Autodesk Inventor part; units mm, degrees
ref_plane "Work Plane1" through (1.525, 0, 0) normal (0, 0, 1) x (1, 0, 0)
ref_plane "YZ Plane" through (0, 0, 0) normal (1, 0, 0) x (0, 1, 0)
ref_plane "XZ Plane" through (0, 0, 0) normal (0, 1, 0) x (-1, 0, 0)
sketch "草图1" plane through (0, 0, 0) normal (0, 0, 1) x (1, 0, 0)
  line L0 (0, 7.25) -> (0, 5)
  line L1 (9, 5) -> (35, 5)
  line L2 (35, 5) -> (35, 0)
  line L3 (35, 0) -> (-0.4001, 0)
  line L4 (-7.4801, 0) -> (42.08, 0)
  line L5 (-0.4001, 0) -> (-0.4001, 7.25)
  line L6 (-0.4001, 7.25) -> (0, 7.25)
  line L7 (9, 5) -> (8.0797, 5)
  line L8 (8.0797, 5) -> (0, 5)
  line L9 (0, -1.45) -> (0, 8.7)
  dimension "d0" = 35
  dimension "d1" = 26
  dimension "d2" = 10
  dimension "d9" = 0.4001
  dimension "d10" = 14.5
  dimension "d13" = 0.9203
  dimension "d14" = 10
revolve "轴承体" add sketch "草图1" angle 360 about axis through (35, 0, 0) along (-1, 0, 0)
sketch "草图2" plane through (-0.4001, 0, 0) normal (-1, 0, 0) x (0, 0, 1)
  line L0 (0, 9.2376) -> (8, 4.6188)
  line L1 (8, 4.6188) -> (8, -4.6188)
  line L2 (8, -4.6188) -> (0, -9.2376)
  line L3 (0, -9.2376) -> (-8, -4.6188)
  line L4 (-8, -4.6188) -> (-8, 4.6188)
  line L5 (-8, 4.6188) -> (0, 9.2376)
  point P0 (0, 0)
  point P1 (0, 0)
  dimension "d11" = 16
extrude "头" add sketch "草图2" along normal blind 6
sketch "草图4" plane through (0, 0, 0) normal (0, 0, 1) x (1, 0, 0)
  line L0 (-6.4001, 8) -> (-6.4001, 9.2376)
  line L1 (-6.4001, 9.2376) -> (-5.6856, 9.2376)
  line L2 (-5.6856, 9.2376) -> (-6.4001, 8)
  line L3 (-7.6001, 0) -> (0.7999, 0)
  line L4 (-0.4001, 9.2376) -> (-6.4001, 9.2376)
  line L5 (-6.4001, 4.6188) -> (-6.4001, 9.2376)
  dimension "d5" = 30
  dimension "d19" = 16
revolve "倒角1" cut sketch "草图4" angle 360 about axis through (-10, 0, 0) along (1, 0, 0)
thread "螺纹"
chamfer "倒角2" distance 0.9202 distance2 0.9203 1 edges at (35, -5, 0) measured on face at (35, -0.8768, 0.3989)
ref_plane "Work Plane1" through (1.525, 0, 0) normal (0, 0, 1) x (1, 0, 0)
equation "\"d11\" = SW"
equation "\"d3\" = KOH - SD"
equation "\"d15\" = GEL"
equation "\"d6\" = -0.5 * SPD + 0.5 * GD"
equation "\"d0\" = NLG"
equation "\"d1\" = GEL"
equation "\"d2\" = GD"
equation "\"d10\" = SD2"
equation "\"d14\" = BDM"
equation "\"d5\" = ANG1"
equation "\"d19\" = SW0"
equation "\"NLG\" = 35"
equation "\"GD\" = NND"
equation "\"BDM\" = NND"
equation "\"KOH\" = 6.4"
equation "\"GEL\" = 26"
equation "\"SW\" = 16"
equation "\"SW0\" = SW"
equation "\"SPD\" = NND - 1.2269 * PTC"
equation "\"SD2\" = SDH"
equation "\"SD\" = WFT"
equation "\"ANG1\" = 30deg"
equation "\"GAL\" = 0.61345 * PTC"
equation "\"GUL\" = 0.61345 * PTC"
equation "\"RR\" = 0.4"
equation "\"WFT\" = 0.4"
equation "\"GD1\" = THREADDIA - 1.2269 * PTC"
equation "\"SDH\" = 14.5"
equation "\"TOA\" = 30deg"
equation "\"FAWI\" = 45deg"
equation "\"PTC\" = 1.5"
equation "\"E0\" = 1.155 * SW"
properties part number "螺栓 GB/T 5782 M10 x 35" material "钢，软"
Geometry check sheet. Reference: the model listing, model coordinates, mm. A direction names the side the tool comes from. Coordinates: 2 decimals unless noted, no trailing zeros. Order: outer loops, then holes, each group sorted by start corner. A loop starts at its lowest first (then second) coordinate and runs counter-clockwise, first axis right, second up. Notation, with made-up numbers: M 58,45 L 67,45 A29 ccw 67,67 Z; hole C 27.5,30.25 d8. An arc over 180 degrees is marked long. One line per question, with ' | ' between items. Start each with the question number.
Item 1: Set-up check for faces 1 (the cylindrical face through (16.8, -1.08, 4.88)), 2 (the conical face through (-6.226, -4.133, 7.199)): record each of +Z, -Z, +X, -X, +Y, -Y from which the full face is reachable in a straight line by a thin tool's end or side.
Item 2: Gauge pin test, flat ends, axial feed: pin 1 (3 mm diameter, centred on y = -3, z = -5, fed in from +X); pin 2 (6 mm diameter, centred on x = 23.5, z = 4, fed in from -Y); pin 3 (1.5 mm diameter, centred on x = 27.5, y = -1, fed in from -Z); pin 4 (6 mm diameter, centred on x = 0.5, y = -0.5, fed in from -Z). Record the tip position at first contact, or that the pin passes through.
Item 3: Material ranges on L1, parallel to X at y = 5.25, z = 5.75; L2, parallel to X at y = 1.25, z = 7; L3, parallel to Z at x = 2, y = 0, recorded low to high. Write a range as [from, to].
Item 4: Cross-section at A-A on x = 3. Enter the section's corners in (y, z), then the cut area to 3 significant figures.
Findings:
1) face 1: +X | face 2: +Z, -X, -Y
2) pin 1: stops at x = 34.75 | pin 2: stops at y = -4.9 | pin 3: stops at z = -4.99 | pin 4: stops at z = -8
3) L1: x = [-6.4, -0.4] | L2: x = [-6.4, 0] | L3: z = [-5, 5]
4) outline: C 0,0 d10 | area: 78.5 mm²
